Design review of the part shown in the three views and the two pictorial views. Dimensions are in mm from the part's minimum x, y and z. A direction names the side the tool comes from. Coordinates: 2 decimals unless noted, no trailing zeros. Loops run counter-clockwise (first coordinate to the right, second up) from the corner with the lowest first, then second, coordinate; pieces in that order, holes last. Notation, with made-up numbers: M 79,-16 L 105,-16 A20 cw 105,-7 Z; hole C -36,86 d8. An arc over 180 degrees is marked long. Answer as a JSON object with one key per item and string values. Group by question number.
Item 1: Add section B-B (x = 31). State the section outline as (y, z) points.
Item 2: Wall thickness on L1, parallel to Y at x = 22.5, z = 8; L2, parallel to X at y = 26.5, z = 1.75; L3, parallel to X at y = 6.5, z = 9: over which ranges is each line inside the solid? List them lowest first. Write a range as from..to.
Item 3: Add section A-A (y = 17). State the section outline as (x, z) points.
Item 4: Add section C-C (z = 1.25). State the section outline as (x, y) points.
Item 5: Mouldability with a two-part tool opening along X and no side actions: class the marked faces 3, 4, 5 and 6 as +X half, -X half, draft (parallel to the pull), parting line (faces both ways), or undercut.
Item 6: Tool access review of the marked faces 1 and 2: name each direction out of +Z, -Z, +X, -X, +Y, -Y from which nothing blocks a thin tool from reaching the whole face with its end or side.
Item 7: Insertion check: pin 1 (12 mm diameter, centred on x = 31.5, y = 29.5, fed in from +Z). The pin has a flat end and moves straight along its axis. Give the tip position at first contact, or say it passes through.
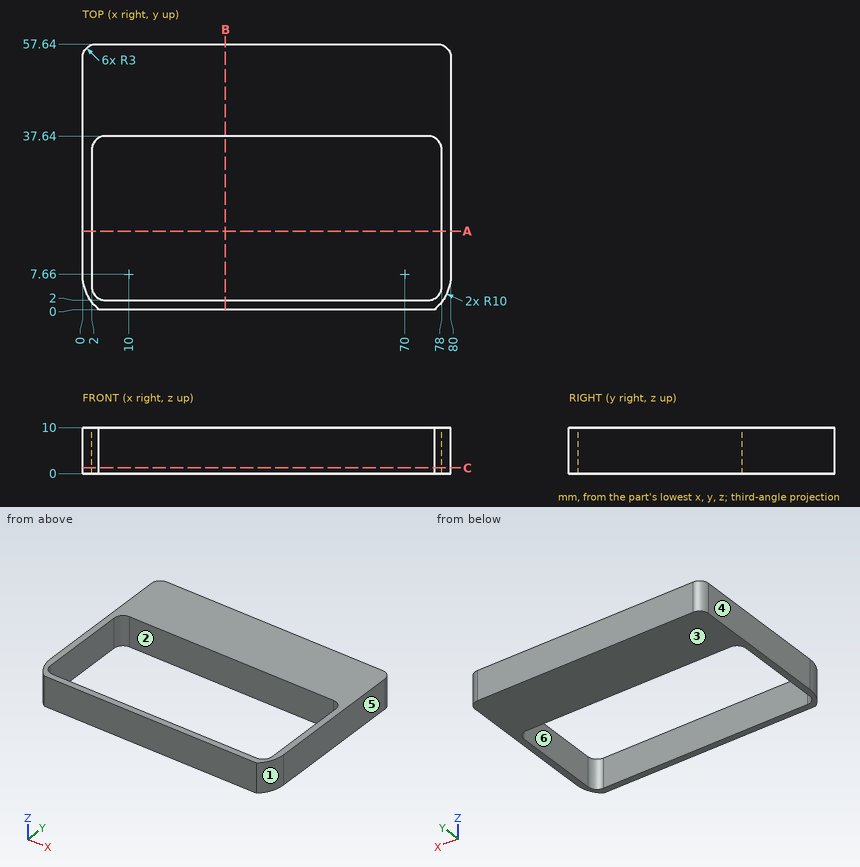
From the geometry:
{
 "1": {"outline": "M 0,0 L 2,0 L 2,10 L 0,10 Z; M 37.64,0 L 57.64,0 L 57.64,10 L 37.64,10 Z"},
 "2": {"L1": "y = 0..2, 37.64..57.64", "L2": "x = 0..2, 78..80", "L3": "x = 0.07..2, 78..79.93"},
 "3": {"outline": "M 0,0 L 2,0 L 2,10 L 0,10 Z; M 78,0 L 80,0 L 80,10 L 78,10 Z"},
 "4": {"outline": "M 0,7.66 A10 ccw 3.57,0 L 76.43,0 A10 ccw 80,7.66 L 80,54.64 A3 ccw 77,57.64 L 3,57.64 A3 ccw 0,54.64 Z; hole M 2,5 A3 ccw 5,2 L 75,2 A3 ccw 78,5 L 78,34.64 A3 ccw 75,37.64 L 5,37.64 A3 ccw 2,34.64 Z"},
 "5": {"face 3": "draft", "face 4": "-X half", "face 5": "+X half", "face 6": "undercut"},
 "6": {"face 1": "+Z, -Z, +X, -Y", "face 2": "+Z, -Z"},
 "7": {"pin 1": "passes through"}
}
